The figure shows three views and two pictorial views of one solid part (mm, origin at its lowest corner). Answer the questions. A direction names the side the tool comes from. Round coordinates to 2 decimals unless told otherwise and drop trailing zeros. Order: outer loops, then holes, each group sorted by start corner. A loop starts at its lowest first (then second) coordinate and runs counter-clockwise, first axis right, second up. Notation, with made-up numbers: (56.25, -29.5) -> (83.25, -29.5) arc R25 cw to (83.25, 6.5) -> close; hole circle Ø10 at (-6.5, -5.5). An arc over 180 degrees is marked (long way). One line per item, written item: value. Start each with the question number.
1. Flat-ended cylindrical pins translate along their axes: pin 1 Ø1.5 at (x, z) = (33.5, 10.5) entering from +Y; pin 2 Ø2 at (y, z) = (11.5, 4.5) entering from -X. Find the tip coordinate at first contact, or state that the pin passes through.
2. The mould has two halves that part along Y. Classify the marked faces 1, 2, 3 and 4: released by +Y, released by -Y, zero draft, split by the parting line, or undercut.
3. Section C-C (z = 12) is taken. Give the vertices of the cut face in (x, y).
4. Section A-A (y = 12.75) is taken. Give the vertices of the cut face in (x, z), then the cut area to 3 significant figures.
5. For the marked faces 5, 6 and 7, determine the directions among +Z, -Z, +X, -X, +Y, -Y from which every point of the face is accessible in a straight line to the end or side of a thin tool.
6. Section D-D (y = 2.5) is taken. Give the vertices of the cut face in (x, z), then the cut area to 3 significant figures.
7. Section B-B (x = 32) is taken. Give the vertices of the cut face in (y, z), then the cut area to 3 significant figures.
8. Consider line 1 (X direction, y = 2, z = 9); line 2 (Y direction, x = 2, z = 3.75); line 3 (Z direction, x = 32, y = 2.15). Determine where each line is inside the solid, lowest interval first.
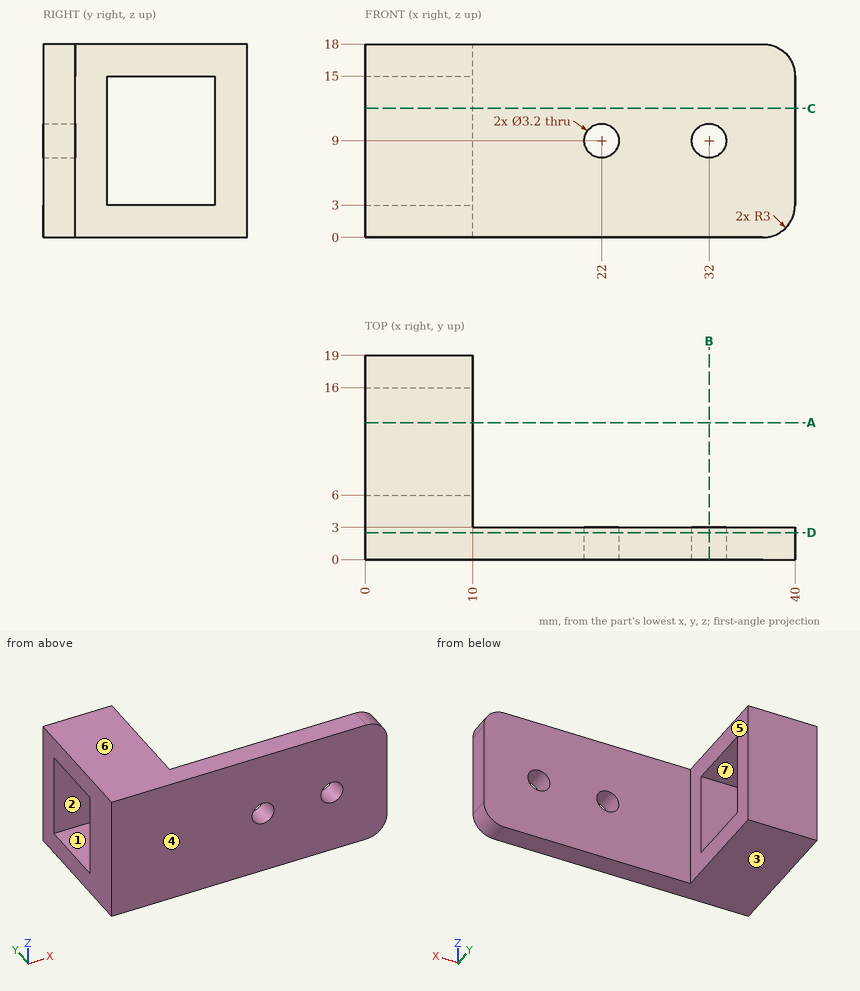
Answer:
1. pin 1: y = 3
1. pin 2: through
2. face 1: undercut
2. face 2: undercut
2. face 3: zero draft
2. face 4: released by -Y
3. outline: (0, 0) -> (40, 0) -> (40, 3) -> (10, 3) -> (10, 6) -> (0, 6) -> close; (0, 16) -> (10, 16) -> (10, 19) -> (0, 19) -> close
4. outline: (0, 0) -> (10, 0) -> (10, 3) -> (0, 3) -> close; (0, 15) -> (10, 15) -> (10, 18) -> (0, 18) -> close
4. area: 60.0 mm^2
5. face 5: +Z, -Z, +X, +Y
5. face 6: +Z, +X, -X, +Y, -Y
5. face 7: +X, -X
6. outline: (0, 0) -> (37, 0) arc R3 ccw to (40, 3) -> (40, 15) arc R3 ccw to (37, 18) -> (0, 18) -> close; hole circle Ø3.2 at (22, 9); hole circle Ø3.2 at (32, 9)
6. area: 700 mm^2
7. outline: (0, 0) -> (3, 0) -> (3, 7.4) -> (0, 7.4) -> close; (0, 10.6) -> (3, 10.6) -> (3, 18) -> (0, 18) -> close
7. area: 44.4 mm^2
8. line 1: 0 to 20.4, 23.6 to 30.4, 33.6 to 40
8. line 2: 0 to 6, 16 to 19
8. line 3: 0 to 7.4, 10.6 to 18
